from build123d import *

# Parameters (mm, degrees)
F1_DEPTH    = 24
F2_T2_ANGLE = 335.5716732895
F2_T4_ANGLE = 335.5716732895
F2_T6_ANGLE = 253.6182255886
F2_T8_ANGLE = 253.6182255886


# Not quite as in the source:
# - a fillet or chamfer that OpenCascade refuses, or shapes differently, is made with other operations: its cross-section is extruded or revolved along the edge and cut away or added


with BuildPart() as f1:
    # F0 (on Front) → F1 (new body)
    with BuildSketch(Plane.XZ):
        with BuildLine():
            Line((1.5, 2), (-1.5, 2))
            ThreePointArc((-1.5, 2), (-2.5, 0), (-1.5, -2))
            Line((-1.5, -2), (1.5, -2))
            ThreePointArc((1.5, -2), (2.5, 0), (1.5, 2))
        make_face()
    extrude(amount=F1_DEPTH)

    # F2: fillet of radius 2 on 4 edges, made by hand

    # F2_s1 → F2_t2 (revolve, cut)
    with BuildSketch(Plane(origin=(0, 0, 0), x_dir=(0, 1, 0), z_dir=(0.2115664045, 0, -0.9773636255))):
        with BuildLine():
            ThreePointArc((-2, 2.5), (-0.5857864376, 1.9142135624), (0, 0.5))
            Line((0, 0.5), (0, 2.5))
            Line((0, 2.5), (-2, 2.5))
        make_face()
    revolve(axis=Axis((0, 0, 0), (0, -1, 0)), revolution_arc=F2_T2_ANGLE, mode=Mode.SUBTRACT)

    # F2_s3 → F2_t4 (revolve, cut)
    with BuildSketch(Plane(origin=(0, 0, 0), x_dir=(0, 1, 0), z_dir=(0.2115664045, 0, -0.9773636255))):
        with BuildLine():
            ThreePointArc((-22, 2.5), (-23.4142135624, 1.9142135624), (-24, 0.5))
            Line((-24, 0.5), (-24, 2.5))
            Line((-24, 2.5), (-22, 2.5))
        make_face()
    revolve(axis=Axis((0, -24, 0), (0, -1, 0)), revolution_arc=F2_T4_ANGLE, mode=Mode.SUBTRACT)

    # F2_s5 → F2_t6 (revolve, cut)
    with BuildSketch(Plane(origin=(0, 0, 0), x_dir=(0, 1, 0), z_dir=(-0.8006360872, 0, 0.5991509459))):
        with BuildLine():
            ThreePointArc((-2, 2.5), (-0.5857864376, 1.9142135624), (0, 0.5))
            Line((0, 0.5), (0, 2.5))
            Line((0, 2.5), (-2, 2.5))
        make_face()
    revolve(axis=Axis((0, 0, 0), (0, -1, 0)), revolution_arc=F2_T6_ANGLE, mode=Mode.SUBTRACT)

    # F2_s7 → F2_t8 (revolve, cut)
    with BuildSketch(Plane(origin=(0, 0, 0), x_dir=(0, 1, 0), z_dir=(-0.8006360872, 0, 0.5991509459))):
        with BuildLine():
            ThreePointArc((-22, 2.5), (-23.4142135624, 1.9142135624), (-24, 0.5))
            Line((-24, 0.5), (-24, 2.5))
            Line((-24, 2.5), (-22, 2.5))
        make_face()
    revolve(axis=Axis((0, -24, 0), (0, -1, 0)), revolution_arc=F2_T8_ANGLE, mode=Mode.SUBTRACT)


solid = f1.part
Input: part model. Units: mm. Frame: model coordinates. Round coordinates to 2 decimals unless told otherwise and drop trailing zeros. Loops run counter-clockwise (first coordinate to the right, second up) from the corner with the lowest first, then second, coordinate; pieces in that order, holes last. Notation, with made-up numbers: (-38, -8) -> (-15, -8) arc R26 ccw to (-15, 18) -> close; hole circle Ø3 at (85, -8.75). An arc over 180 degrees is marked (long way). Answer as a JSON object with one key per item and string values. Group by question number.
1) Pin query (flat end, axial travel): pin 1 (1 mm diameter, centred on y = -12.5, z = 1, fed in from +X). Return the tip coordinate at first contact, or that it passes through.
2) Ray query, L1, parallel to Z at x = 2, y = -19; L2, parallel to Y at x = -0.1, z = -1.15; L3, parallel to X at y = -22.75, z = -1.6. Return the intervals inside material, ascending.
3) Section query A-A on y = -5.25. Output: boundary loops of the cut face in (x, z).
Reply:
{
 "1": {"pin 1": "stops at x = 2.45"},
 "2": {"L1": "z = -1.5 to 1.5", "L2": "y = -23.89 to -0.11", "L3": "x = -1.73 to 1.73"},
 "3": {"outline": "(-1.5, -2) -> (1.5, -2) arc R2.5 ccw to (1.5, 2) -> (-1.5, 2) arc R2.5 ccw to start"}
}
